Could you check a few things on this model? Use its own coordinates, in mm. Coordinates: 2 decimals unless noted, no trailing zeros. Order: outer loops, then holes, each group sorted by start corner. A loop starts at its lowest first (then second) coordinate and runs counter-clockwise, first axis right, second up. Notation, with made-up numbers: (-1.5, -32) -> (40.5, -32) arc R26 cw to (40.5, -1) -> close; hole circle Ø10 at (14.5, 71.5). An arc over 180 degrees is marked (long way). Put each result on its own line as item: value. Start each with the question number.
Q1. If we section it at B-B (z = 21): Please give me the cut outline in (x, y), and give its area (3 significant figures).
Q2. Will these pins go through, and if not, where does the flat tip stop? pin 1 (2 mm diameter, centred on x = 30.5, y = 0.5, fed in from +Z); pin 2 (1 mm diameter, centred on x = -0.5, y = 1, fed in from +Z).
Q3. We'd pull the mould along X, two halves only. Please class faces 1 (the face through (1.168, -1.074, -55.038)), 2 (the face through (94.333, 0.078, 0.612)): +X half, -X half, draft (parallel to the pull), parting line (faces both ways), or undercut.
Q4. If we section it at A-A (y = 0): Please give me the cut outline in (x, z).
Q5. If we section it at C-C (x = 81): Please give me the cut outline in (y, z).
Q6. Please list where these lines run through material, in increasing order: line 1 along X through (y, z) = (-0.1, 4); line 2 along X through (y, z) = (0.3, -19); line 3 along Z through (x, y) = (5.5, 1.15).
from build123d import *

# Parameters (mm, degrees)
O_RINGPROFILE_R = 1.7653


with BuildPart() as part:
    # Sweep2: sweep along a path in O-RingPath
    with BuildLine(Plane(origin=(0, 0, 0), x_dir=(1, 0, 0), z_dir=(0, 1, 0))) as sweep2_path:
        Line((83.396775144, -56.4388), (-83.396775144, -56.4388))
        ThreePointArc((-83.396775144, -56.4388), (-92.377031265, -52.719056121), (-96.096775144, -43.7388))
        Line((-96.096775144, -43.7388), (-96.096775144, 43.7388))
        ThreePointArc((-96.096775144, 43.7388), (-92.377031265, 52.719056121), (-83.396775144, 56.4388))
        Line((-83.396775144, 56.4388), (83.396775144, 56.4388))
        ThreePointArc((83.396775144, 56.4388), (92.377031265, 52.719056121), (96.096775144, 43.7388))
        Line((96.096775144, 43.7388), (96.096775144, -43.7388))
        ThreePointArc((96.096775144, -43.7388), (92.377031265, -52.719056121), (83.396775144, -56.4388))
    # O-RingProfile → Sweep2 (sweep)
    with BuildSketch(Plane.XY):
        with Locations((96.096775144, 0)):
            Circle(O_RINGPROFILE_R)
    sweep(path=sweep2_path.line)


solid = part.part
The answers:
1. outline: circle Ø3.53 at (-96.1, 0); circle Ø3.53 at (96.1, 0)
1. area: 19.6 mm^2
2. pin 1: z = 58.2
2. pin 2: z = 58.13
3. face 1: undercut
3. face 2: undercut
4. outline: (-97.86, -43.74) arc R14.47 ccw to (-83.4, -58.2) -> (83.4, -58.2) arc R14.47 ccw to (97.86, -43.74) -> (97.86, 43.74) arc R14.47 ccw to (83.4, 58.2) -> (-83.4, 58.2) arc R14.47 ccw to (-97.86, 43.74) -> close; hole (-94.33, -43.74) arc R10.93 ccw to (-83.4, -54.67) -> (83.4, -54.67) arc R10.93 ccw to (94.33, -43.74) -> (94.33, 43.74) arc R10.93 ccw to (83.4, 54.67) -> (-83.4, 54.67) arc R10.93 ccw to (-94.33, 43.74) -> close
5. outline: circle Ø3.53 at (0, -56.44); circle Ø3.53 at (0, 56.44)
6. line 1: -97.86 to -94.33, 94.33 to 97.86
6. line 2: -97.84 to -94.36, 94.36 to 97.84
6. line 3: -57.78 to -55.1, 55.1 to 57.78
